from build123d import *

# Parameters (mm, degrees)
SKETCH_2_R      = 17.5
EXTRUDE_1_DEPTH = 114.7
SKETCH_3_R      = 10.5
SKETCH_3_R_2    = 9.5
EXTRUDE_2_DEPTH = 1.4
EXTRUDE_6_DEPTH = 15.3
SKETCH_8_W      = 2.7
SKETCH_8_H      = 2.7
EXTRUDE_7_DEPTH = 8
SKETCH_8_3_W    = 0.7
SKETCH_8_3_H    = 0.7
EXTRUDE_8_DEPTH = 2


with BuildPart() as part:
    # 草图2 → 凸台-拉伸1 (new body)
    with BuildSketch(Plane(origin=(0, 0, 0), x_dir=(0, 0, -1), z_dir=(1, 0, 0))):
        Circle(SKETCH_2_R)
    extrude(amount=EXTRUDE_1_DEPTH)

    # 草图3 → 凸台-拉伸2 (add)
    with BuildSketch(Plane(origin=(114.7, 0, 0), x_dir=(0, 0, -1), z_dir=(1, 0, 0))):
        Circle(SKETCH_3_R)
        Circle(SKETCH_3_R_2, mode=Mode.SUBTRACT)
    extrude(amount=EXTRUDE_2_DEPTH)

    # 草图6 → 凸台-拉伸6 (add)
    with BuildSketch(Plane.ZY):
        with BuildLine():
            Line((-15.2, 0), (-15.2, -25.2))
            Line((-15.2, -25.2), (15.2, -25.2))
            Line((15.2, -25.2), (15.2, 0))
            ThreePointArc((15.2, 0), (0, 15.2), (-15.2, 0))
        make_face()
    extrude(amount=EXTRUDE_6_DEPTH)

    # 草图8 → 凸台-拉伸7 (add)
    with BuildSketch(Plane.XZ.offset(25.2)):
        with Locations((-5.65, -4.25)):
            Rectangle(SKETCH_8_W, SKETCH_8_H)
        with Locations((-5.65, 1.15)):
            Rectangle(SKETCH_8_W, SKETCH_8_H)
        with Locations((-5.65, 6.55)):
            Rectangle(SKETCH_8_W, SKETCH_8_H)
    extrude(amount=EXTRUDE_7_DEPTH)

    # 草图8<3> → 凸台-拉伸8 (add)
    with BuildSketch(Plane.XZ.offset(25.2)):
        with Locations((-5.65, -1.55)):
            Rectangle(SKETCH_8_3_W, SKETCH_8_3_H)
        with Locations((-5.65, 3.85)):
            Rectangle(SKETCH_8_3_W, SKETCH_8_3_H)
    extrude(amount=EXTRUDE_8_DEPTH)


solid = part.part
CAD build for the part. Positions are in the model's coordinates, mm. A direction names the side the tool comes from. Give positions to 0.01 mm unless a question says otherwise; leave off trailing zeros. Order: outer loops, then holes, each group sorted by start corner. A loop starts at its lowest first (then second) coordinate and runs counter-clockwise, first axis right, second up. Notation, with made-up numbers: (51, 76.5) - (62, 76.5) arc R26 ccw to (62, 90.5) - close; hole circle Ø9 at (17, 75). An arc over 180 degrees is marked (long way). Answer in a Markdown table with one row per item.
1. Saw through at A-A, the plane y = 4.5. Give the cut face in (x, z).
Data:
| item | result |
|---|---|
| outline | (-15.3, -14.52) - (0, -14.52) - (0, -16.91) - (114.7, -16.91) - (114.7, -9.49) - (116.1, -9.49) - (116.1, -8.37) - (114.7, -8.37) - (114.7, 8.37) - (116.1, 8.37) - (116.1, 9.49) - (114.7, 9.49) - (114.7, 16.91) - (0, 16.91) - (0, 14.52) - (-15.3, 14.52) - close |
2. Tool access for faces 4 (the cylindrical face through (-7.543, 15.196, 0.334)), 5 (the flat face through (114.7, -8, -8)), 6 (the flat face through (-8, -12, -15.2)), 7 (the flat face through (-6, -29, 5.2)), 8 (the flat face through (-7, -29, 7)): list every direction of +Z, -Z, +X, -X, +Y, -Y with a clear straight run to the whole face (end or side of a thin tool).
Data:
| item | result |
|---|---|
| face 4 | -X, +Y |
| face 5 | +X |
| face 6 | -Z, -X, +Y, -Y |
| face 7 | +X, -X, -Y |
| face 8 | +Z, -Z, -X, -Y |
3. Probe probe 1 along Y at (x, z) = (115.1, 0); probe 2 along X at (y, z) = (-9, 6.5); probe 3 along X at (y, z) = (-20, -7.5). List the from-to ranges inside material, lowest first. Write a range as [from, to].
Data:
| item | result |
|---|---|
| probe 1 | y = [-10.5, -9.5], [9.5, 10.5] |
| probe 2 | x = [-15.3, 114.7] |
| probe 3 | x = [-15.3, 0] |
4. Saw through at D-D, the plane y = -13. Give the cut face in (x, z).
Data:
| item | result |
|---|---|
| outline | (-15.3, -15.2) - (0, -15.2) - (0, -11.72) - (114.7, -11.72) - (114.7, 11.72) - (0, 11.72) - (0, 15.2) - (-15.3, 15.2) - close |
5. Flat gauge pins, fed straight in: pin 1 (8 mm diameter, centred on x = 7, z = -3, fed in from +Y); pin 2 (1.4 mm diameter, centred on y = -29, z = 1.5, fed in from -X); pin 3 (0.6 mm diameter, centred on x = -5.5, z = -1.5, fed in from -Y); pin 4 (0.6 mm diameter, centred on y = -26, z = 4, fed in from +X). Where does each tip first touch, or does it go through?
Data:
| item | result |
|---|---|
| pin 1 | stops at y = 17.5 |
| pin 2 | stops at x = -7 |
| pin 3 | stops at y = -27.2 |
| pin 4 | stops at x = -5.3 |
6. Pull direction Y, two halves, no side cores. Call faces 1 (the flat face through (-6, -29, 7.9)), 2 (the cylindrical face through (56.547, -10.648, 13.887)), 3 (the flat face through (114.7, 0, 0)): pulls with the +Y half, pulls with the -Y half, needs draft (parallel to the pull), parting line crosses it, or undercut.
Data:
| item | result |
|---|---|
| face 1 | needs draft |
| face 2 | parting line crosses it |
| face 3 | undercut |
7. Saw through at B-B, the plane z = -8. Give the cut face in (x, y), plus the area to 3 significant figures.
Data:
| item | result |
|---|---|
| outline | (-15.3, -25.2) - (0, -25.2) - (0, -15.56) - (114.7, -15.56) - (114.7, -6.8) - (116.1, -6.8) - (116.1, -5.12) - (114.7, -5.12) - (114.7, 5.12) - (116.1, 5.12) - (116.1, 6.8) - (114.7, 6.8) - (114.7, 15.56) - (0, 15.56) - (0, 12.92) - (-15.3, 12.92) - close |
| area | 4,160 mm² |
8. Saw through at C-C, the plane x = 66. Give the cut face in (y, z).
Data:
| item | result |
|---|---|
| outline | circle Ø35 at (0, 0) |
